Part model, mm, in its own coordinate system. A direction names the side the tool comes from. Coordinates: 2 decimals unless noted, no trailing zeros. Loops run counter-clockwise (first coordinate to the right, second up) from the corner with the lowest first, then second, coordinate; pieces in that order, holes last. Notation, with made-up numbers: M 10.5,21 L 14.5,21 A24 cw 14.5,48 Z; hole C 59.5,16 d11. An arc over 180 degrees is marked long. Use CSV: the item, a comma, the result in double quotes. Start each with the question number.
from build123d import *

# Parameters (mm, degrees)
F1_DEPTH = 10
F3_DEPTH = 5


# Not quite as in the source:
# - a feature names something its author has since deleted; it is built from what else it names


with BuildPart() as f1:
    # F0 (on Front) → F1 (new body)
    with BuildSketch(Plane.XZ):
        with BuildLine():
            Line((4.5435639801, -4.8811539246), (47.0578219503, -4.8811539246))
            Line((47.0578219503, -4.8811539246), (47.0578219503, 5.1188460754))
            ThreePointArc((47.0578219503, 5.1188460754), (13.0237482483, 31.7276460361), (-16.4989304836, 0.1878640363))
            ThreePointArc((-16.4989304836, 0.1878640363), (-13.5129700245, -9.4683494399), (-5.4564360199, -15.5716828237))
            Line((-5.4564360199, -15.5716828237), (-5.4564360199, -46.8141730692))
            Line((-5.4564360199, -46.8141730692), (4.5435639801, -46.8141730692))
            Line((4.5435639801, -46.8141730692), (4.5435639801, -4.8811539246))
        make_face()
    extrude(amount=F1_DEPTH)

    # F2 (on face) → F3 (cut)
    with BuildSketch(Plane.XZ.offset(10)):
        Polygon((47.0578219503, -2.6311539246), (47.0578219503, 2.8688460754), (-3.2064360199, 2.8688460754), (-3.2064360199, -2.6311539246), (-3.2064360199, -46.8141730692), (2.2935639801, -46.8141730692), (2.2935639801, -2.6311539246), align=None)
    extrude(amount=-F3_DEPTH, mode=Mode.SUBTRACT)


solid = f1.part
1. Tool access for faces 1 (the face through (4.544, -5, -26)), 2 (the face through (-5.456, -5, -31)), 3 (the face through (47.058, -4, 0)), 4 (the face through (13.686, -4.93, 31.772)), 5 (the face through (-3.206, -8, -22)): list every direction of +Z, -Z, +X, -X, +Y, -Y with a clear straight run to the whole face (end or side of a thin tool).
2. Wall check: probe 1 along X at (y, z) = (-1.75, -17); probe 2 along X at (y, z) = (-5.75, -5); probe 3 along Y at (x, z) = (-3, -24). Give the ranges that are in metal, low to high.
3. Slice it at B-B, the plane y = -3.5. List the corners of the cut face in (x, z), and give its area (3 significant figures).
4. Two-plate mould, pull along Z, no slides. Class faces 6 (the face through (2.294, -8, -25)), 7 (the face through (22, -8, 2.869)), 8 (the face through (24, -8, -2.631)), 9 (the face through (-1, -4, -46.814)): pulls with the +Z half, pulls with the -Z half, needs draft (parallel to the pull), parting line crosses it, or undercut.
5. Slice it at C-C, the plane z = -38.5. List the corners of the cut face in (x, y), and give its area (3 significant figures).
6. Pin check, flat tips, straight feed: pin 1 (4 mm diameter, centred on x = 28.5, y = -8.5, fed in from +Z); pin 2 (3 mm diameter, centred on y = -6.5, z = -25, fed in from -X); pin 3 (10 mm diameter, centred on x = 35, z = -0.5, fed in from -Y); pin 4 (4 mm diameter, centred on y = -8, z = -23.5, fed in from +X). Stop position of each tip, or through.
7. Slice it at D-D, the plane x = 35. List the corners of the cut face in (y, z), and give its area (3 significant figures).
8. Slice it at A-A, the plane y = -8.75. List the corners of the cut face in (x, z), and give its area (3 significant figures).
Found:
1,face 1,"-Z, +X, +Y, -Y"
1,face 2,"-Z, -X, +Y, -Y"
1,face 3,"+Z, -Z, +X, +Y, -Y"
1,face 4,"+Z, +Y, -Y"
1,face 5,"-Z, -Y"
2,probe 1,"-5.46 to 4.54"
2,probe 2,"-15.72 to -3.21, 2.29 to 4.54"
2,probe 3,"-5 to 0"
3,outline,"M -16.5,0.19 A16.5 ccw -5.46,-15.57 L -5.46,-46.81 L 4.54,-46.81 L 4.54,-4.88 L 47.06,-4.88 L 47.06,5.12 A32 ccw Z"
3,area,"2,400 mm^2"
4,face 6,"needs draft"
4,face 7,"undercut"
4,face 8,"undercut"
4,face 9,"pulls with the -Z half"
5,outline,"M -5.46,-10 L -3.21,-10 L -3.21,-5 L 2.29,-5 L 2.29,-10 L 4.54,-10 L 4.54,0 L -5.46,0 Z"
5,area,"72.5 mm^2"
6,pin 1,"z = 29.87"
6,pin 2,"x = -5.46"
6,pin 3,"y = -10"
6,pin 4,"x = 4.54"
7,outline,"M -10,-4.88 L 0,-4.88 L 0,25.19 L -10,25.19 L -10,2.87 L -5,2.87 L -5,-2.63 L -10,-2.63 Z"
7,area,"273 mm^2"
8,outline,"M -16.5,0.19 A16.5 ccw -5.46,-15.57 L -5.46,-46.81 L -3.21,-46.81 L -3.21,2.87 L 47.06,2.87 L 47.06,5.12 A32 ccw Z; M 2.29,-46.81 L 4.54,-46.81 L 4.54,-4.88 L 47.06,-4.88 L 47.06,-2.63 L 2.29,-2.63 Z"
8,area,"1,880 mm^2"
